Autodesk Inventor part; units mm, degrees
ref_plane "YZ Plane" through (0, 0, 0) normal (1, 0, 0) x (0, 1, 0)
ref_plane "XZ Plane" through (0, 0, 0) normal (0, 1, 0) x (-1, 0, 0)
ref_plane "XY Plane" through (0, 0, 0) normal (0, 0, 1) x (1, 0, 0)
sketch "草圖1" plane through (0, 0, 0) normal (0, 0, 1) x (1, 0, 0)
  arc A0 (-17.5, 0) -> (17.5, 0) centre (0, 0) ccw
  arc A1 (-20, 0) -> (20, 0) centre (0, 0) ccw
  line L0 (-20, 0) -> (-17.5, 0)
  line L1 (20, 0) -> (17.5, 0)
  line L2 (-35, 0) -> (35, 0)
  line L3 (-25, 0) -> (25, 0)
  line L4 (25, -65) -> (-25, -65)
  line L5 (-25, -65) -> (-25, 0)
  line L6 (-25, 0) -> (25, 0)
  line L7 (25, 0) -> (25, -65)
  line L8 (25, -65) -> (-25, 0) construction
  line L9 (-25, -65) -> (25, 0) construction
  line L10 (0, -78) -> (0, 13)
  point P0 (17.5, 0)
  point P1 (20, 0)
  point P2 (20, 0)
  point P3 (0, -32.5)
  dimension "d0" = 17.5
  dimension "d16" = 50
  dimension "d17" = 65
  dimension "d22" = 20
extrude "擠出1" add sketch "草圖1" along normal mid plane 20 contours L2 L10 A0 | A0 L10 A1 L0 | L10 L2 A0 | A0 L1 A1 L10
extrude "擠出2" add sketch "草圖1" along normal mid plane 5
sketch "草圖2" plane through (0, 0, 0) normal (1, 0, 0) x (0, 1, 0)
  line L0 (-10, -10) -> (-5, 10)
  line L1 (0, -2.5) -> (0, -10)
  line L2 (0, 10) -> (0, 2.5)
  line L3 (-20, -10) -> (0, -10)
  line L4 (0, 10) -> (-20, 10)
  point P0 (0, 0)
  dimension "d18" = 10
  dimension "d19" = 5
sketch "草圖3" plane through (0, 0, -10) normal (0, 0, -1) x (-1, 0, 0)
  arc A0 (-17.5, 0) -> (17.5, 0) centre (0, 0) ccw
  line L0 (25, 0) -> (-25, 0)
sweep "掃掠1" cut profiles "草圖3" path "草圖2" path curves L0
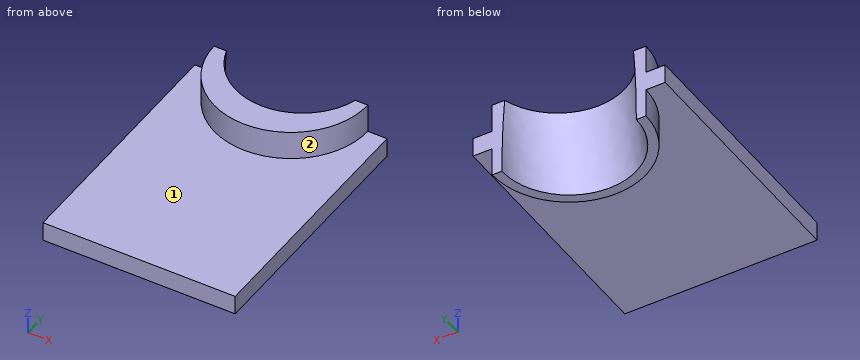
Model file for the job. Use its own axes, mm. Face numbers are marked on the shaded views. Give positions to 0.01 mm unless a question says otherwise; leave off trailing zeros. Order: outer loops, then holes, each group sorted by start corner. A loop starts at its lowest first (then second) coordinate and runs counter-clockwise, first axis right, second up. Notation, with made-up numbers: (61, 34) - (91, 34) arc R13 ccw to (91, 46) - close; hole circle Ø6 at (44, -8). An arc over 180 degrees is marked (long way). One line per item, written item: value.
Item 1: Pin check, flat tips, straight feed: pin 1 Ø12 at (x, y) = (-1.5, -34.5) entering from +Z; pin 2 Ø5 at (x, y) = (9.5, -33.5) entering from -Z; pin 3 Ø1 at (y, z) = (-9, 6.5) entering from +X; pin 4 Ø6 at (y, z) = (-48, -6) entering from -X. Stop position of each tip, or through.
Response values:
pin 1: z = 2.5
pin 2: z = -2.5
pin 3: x = 18.1
pin 4: through
Item 2: Wall check: line 1 (Z direction, x = 14, y = -15.5); line 2 (X direction, y = -4, z = 7.5); line 3 (X direction, y = -5, z = -6.25). Give the ranges that are in metal, low to high.
Response values:
line 1: -2.5 to 2.5
line 2: -19.6 to -15.37, 15.37 to 19.6
line 3: -19.36 to -16.46, 16.46 to 19.36
Item 3: Two-plate mould, pull along X, no slides. Class the marked faces 1 and 2: released by +X, released by -X, zero draft, split by the parting line, or undercut.
Response values:
face 1: zero draft
face 2: split by the parting line
Item 4: Slice it at A-A (y = -40.5). List the corners of the cut face in (x, z).
Response values:
outline: (-25, -2.5) - (25, -2.5) - (25, 2.5) - (-25, 2.5) - close
